Autodesk Inventor part; units mm, degrees
ref_plane "YZ Plane" through (0, 0, 0) normal (1, 0, 0) x (0, 1, 0)
ref_plane "XZ Plane" through (0, 0, 0) normal (0, 1, 0) x (-1, 0, 0)
ref_plane "XY Plane" through (0, 0, 0) normal (0, 0, 1) x (1, 0, 0)
sketch "Skizze1" plane through (0, 0, 0) normal (0, 0, 1) x (1, 0, 0)
  circle A0 centre (0, 0) radius 2.75
  dimension "d0" = 5.5
extrude "Extrusion1" add sketch "Skizze1" along normal blind 3
fillet "Rundung1" radius 2 1 edges at (-2.75, 0, 3)
sketch "Skizze2" plane through (0, 0, 3) normal (0, 0, 1) x (1, 0, 0)
  line L0 (0.25, -2.25) -> (-0.25, -2.25)
  line L1 (-0.25, 2.25) -> (0.25, 2.25)
  line L2 (0.25, -2.25) -> (-0.25, 2.25) construction
  line L3 (-0.25, -2.25) -> (0.25, 2.25) construction
  line L4 (-2.25, 0.25) -> (-2.25, -0.25)
  line L5 (2.25, -0.25) -> (2.25, 0.25)
  line L6 (2.25, 0.25) -> (-2.25, -0.25) construction
  line L7 (-2.25, 0.25) -> (2.25, -0.25) construction
  line L8 (-0.25, 0.25) -> (-2.25, 0.25)
  line L9 (-0.25, 0.25) -> (-0.25, 2.25)
  line L10 (-0.25, -2.25) -> (-0.25, -0.25)
  line L11 (-0.25, -0.0278) -> (-0.25, 0.0278)
  line L12 (2.25, 0.25) -> (0.25, 0.25)
  line L13 (0.0278, 0.25) -> (-0.0278, 0.25)
  line L14 (0.25, -0.25) -> (2.25, -0.25)
  line L15 (-2.25, -0.25) -> (-0.25, -0.25)
  line L16 (-0.0278, -0.25) -> (0.0278, -0.25)
  line L17 (0.25, -0.25) -> (0.25, -2.25)
  line L18 (0.25, 2.25) -> (0.25, 0.25)
  line L19 (0.25, 0.0278) -> (0.25, -0.0278)
  point P0 (0, 0)
  dimension "d4" = 0.5
  dimension "d5" = 4.5
  dimension "d6" = 4.5
  dimension "d7" = 0.5
extrude "Extrusion2" cut sketch "Skizze2" against normal blind 1.5
sketch "Skizze3" plane through (0, 0, 0) normal (0, 0, -1) x (-1, 0, 0)
  circle A0 centre (0, 0) radius 1.5
  dimension "d10" = 3
extrude "Extrusion3" add sketch "Skizze3" along normal blind 8
thread "Gewinde1"
properties part number "M3 Schraube"
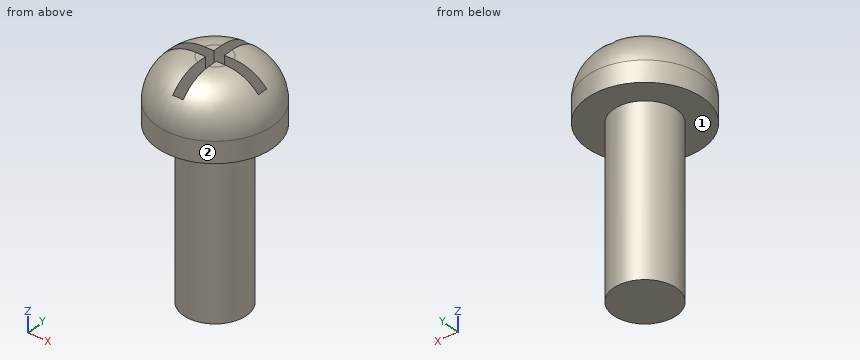
Could you check a few things on this model? Use its own coordinates, in mm. Face numbers are marked on the shaded views. A direction names the side the tool comes from. Round coordinates to 2 decimals unless told otherwise and drop trailing zeros. Loops run counter-clockwise (first coordinate to the right, second up) from the corner with the lowest first, then second, coordinate; pieces in that order, holes last. Notation, with made-up numbers: M 67,3.5 L 102,3.5 A20 ccw 102,10.5 Z; hole C 77.25,22 d5. An arc over 180 degrees is marked long. Write item = value, one per line.
1. Which directions (+Z, -Z, +X, -X, +Y, -Y) give clear straight access to the entire face, cutting with the end or side of a thin tool? Please do the marked faces 1 and 2.
Results below:
face_1 = -Z
face_2 = +Z, -Z
2. I need wall thicknesses on probe 1 along Z at (x, y) = (-1.3, 0.15); probe 2 along Y at (x, z) = (0.35, -7.5); probe 3 along X at (y, z) = (0.1, -2.5). Which ranges of each line are inside material? Lowest first, please.
Results below:
probe_1 = -8 to 1.5
probe_2 = -1.46 to 1.46
probe_3 = -1.5 to 1.5
3. Will these pins go through, and if not, where does the flat tip stop? P1, Ø1.7, axis at y = -1, z = 2, coming from the +X side; P2, Ø0.5, axis at x = 1, z = 2, coming from the -Y side; P3, Ø0.6, axis at y = 0, z = 2, coming from the -X side.
Results below:
P1 = 2.68
P2 = -2.44
P3 = -2.62
4. I want a section at A-A, the plane z = -2.25. Write out the boundary of the cut face in (x, y), and give its area (3 significant figures).
Results below:
outline = C 0,0 d3
area = 7.07 mm²
